from build123d import *

# Parameters (mm, degrees)
BOSS_EXTRU_3_DEPTH = 2
BOSS_EXTRU_4_DEPTH = 19.3
ESQUISSE4_W        = 2
ESQUISSE4_H        = 18.565
ESQUISSE4_H_2      = 18.45
BOSS_EXTRU_5_DEPTH = 3.9
ESQUISSE5_W        = 4
ESQUISSE5_H        = 4
ESQUISSE5_R        = 1.15
ESQUISSE5_W_2      = 3.87
ESQUISSE5_H_2      = 3.3
BOSS_EXTRU_6_DEPTH = 5.7


with BuildPart() as part:
    # Esquisse1 → Boss.-Extru.3 (new body)
    with BuildSketch(Plane.XY):
        with BuildLine():
            Line((-70, 0), (-10.000000065, 0))
            ThreePointArc((-10.000000065, 0), (-2.928932211, 2.928932165), (0, 10))
            Line((0, 10), (0, 110))
            ThreePointArc((0, 110), (-2.928932188, 117.071067812), (-10, 120))
            Line((-10, 120), (-70, 120))
            ThreePointArc((-70, 120), (-77.071067812, 117.071067812), (-80, 110))
            Line((-80, 110), (-80, 10))
            ThreePointArc((-80, 10), (-77.071067812, 2.928932188), (-70, 0))
        make_face()
    extrude(amount=BOSS_EXTRU_3_DEPTH)

    # Esquisse3 → Boss.-Extru.4 (add)
    with BuildSketch(Plane.XY.offset(2)):
        with BuildLine():
            ThreePointArc((-80, 10), (-79.486832981, 6.83772234), (-78, 4))
            Line((-78, 4), (-78, 10))
            Line((-78, 10), (-78, 16))
            ThreePointArc((-78, 16), (-79.486832981, 13.16227766), (-80, 10))
        make_face()
        with BuildLine():
            ThreePointArc((-78, 4), (-77.071067812, 2.928932188), (-76, 2))
            Line((-76, 2), (-70, 2))
            ThreePointArc((-70, 2), (-75.656854249, 4.343145751), (-78, 10))
            Line((-78, 10), (-78, 4))
        make_face()
        with BuildLine():
            ThreePointArc((-76, 2), (-73.16227766, 0.513167019), (-70, 0))
            ThreePointArc((-70, 0), (-66.83772234, 0.513167019), (-64, 2))
            Line((-64, 2), (-70, 2))
            Line((-70, 2), (-76, 2))
        make_face()
        with BuildLine():
            Line((-70, 0), (-10, 0))
            ThreePointArc((-10, 0), (-13.16227766, 0.513167019), (-16, 2))
            Line((-16, 2), (-64, 2))
            ThreePointArc((-64, 2), (-66.83772234, 0.513167019), (-70, 0))
        make_face()
        with BuildLine():
            ThreePointArc((-80, 10), (-79.486832981, 13.16227766), (-78, 16))
            Line((-78, 16), (-78, 104))
            ThreePointArc((-78, 104), (-79.486832981, 106.83772234), (-80, 110))
            Line((-80, 110), (-80, 10))
        make_face()
        with BuildLine():
            ThreePointArc((-80, 110), (-79.486832981, 106.83772234), (-78, 104))
            Line((-78, 104), (-78, 110))
            Line((-78, 110), (-78, 116))
            ThreePointArc((-78, 116), (-79.486832981, 113.16227766), (-80, 110))
        make_face()
        with BuildLine():
            ThreePointArc((-78, 110), (-75.656854249, 115.656854249), (-70, 118))
            Line((-70, 118), (-76, 118))
            ThreePointArc((-76, 118), (-77.071067812, 117.071067812), (-78, 116))
            Line((-78, 116), (-78, 110))
        make_face()
        with BuildLine():
            Line((-70, 118), (-64, 118))
            ThreePointArc((-64, 118), (-66.83772234, 119.486832981), (-70, 120))
            ThreePointArc((-70, 120), (-73.16227766, 119.486832981), (-76, 118))
            Line((-76, 118), (-70, 118))
        make_face()
        with BuildLine():
            Line((-64, 118), (-16, 118))
            ThreePointArc((-16, 118), (-13.16227766, 119.486832981), (-10, 120))
            Line((-10, 120), (-70, 120))
            ThreePointArc((-70, 120), (-66.83772234, 119.486832981), (-64, 118))
        make_face()
        with BuildLine():
            ThreePointArc((-10, 120), (-13.16227766, 119.486832981), (-16, 118))
            Line((-16, 118), (-10, 118))
            Line((-10, 118), (-4, 118))
            ThreePointArc((-4, 118), (-6.83772234, 119.486832981), (-10, 120))
        make_face()
        with BuildLine():
            Line((-2, 110), (-2, 116))
            ThreePointArc((-2, 116), (-2.928932188, 117.071067812), (-4, 118))
            Line((-4, 118), (-10, 118))
            ThreePointArc((-10, 118), (-4.343145751, 115.656854249), (-2, 110))
        make_face()
        with BuildLine():
            ThreePointArc((-2, 104), (-0.513167019, 106.83772234), (0, 110))
            ThreePointArc((0, 110), (-0.513167019, 113.16227766), (-2, 116))
            Line((-2, 116), (-2, 110))
            Line((-2, 110), (-2, 104))
        make_face()
        with BuildLine():
            ThreePointArc((-2, 16), (-0.513167019, 13.16227766), (0, 10))
            Line((0, 10), (0, 110))
            ThreePointArc((0, 110), (-0.513167019, 106.83772234), (-2, 104))
            Line((-2, 104), (-2, 16))
        make_face()
        with BuildLine():
            Line((-2, 10), (-2, 4))
            ThreePointArc((-2, 4), (-0.513167019, 6.83772234), (0, 10))
            ThreePointArc((0, 10), (-0.513167019, 13.16227766), (-2, 16))
            Line((-2, 16), (-2, 10))
        make_face()
        with BuildLine():
            Line((-10, 2), (-4, 2))
            ThreePointArc((-4, 2), (-2.928932188, 2.928932188), (-2, 4))
            Line((-2, 4), (-2, 10))
            ThreePointArc((-2, 10), (-4.343145751, 4.343145751), (-10, 2))
        make_face()
        with BuildLine():
            ThreePointArc((-10, 0), (-6.83772234, 0.513167019), (-4, 2))
            Line((-4, 2), (-10, 2))
            Line((-10, 2), (-16, 2))
            ThreePointArc((-16, 2), (-13.16227766, 0.513167019), (-10, 0))
        make_face()
    extrude(amount=BOSS_EXTRU_4_DEPTH)

    # Esquisse4 → Boss.-Extru.5 (add)
    with BuildSketch(Plane.XY.offset(21.3)):
        with BuildLine():
            Line((-64, 118), (-16, 118))
            ThreePointArc((-16, 118), (-13.16227766, 119.486832981), (-10, 120))
            Line((-10, 120), (-70, 120))
            ThreePointArc((-70, 120), (-66.83772234, 119.486832981), (-64, 118))
        make_face()
        with BuildLine():
            Line((-70, 118), (-64, 118))
            ThreePointArc((-64, 118), (-66.83772234, 119.486832981), (-70, 120))
            ThreePointArc((-70, 120), (-77.071067812, 117.071067812), (-80, 110))
            ThreePointArc((-80, 110), (-79.486832981, 106.83772234), (-78, 104))
            Line((-78, 104), (-78, 110))
            ThreePointArc((-78, 110), (-75.656854249, 115.656854249), (-70, 118))
        make_face()
        with BuildLine():
            Line((-2, 110), (-2, 104))
            ThreePointArc((-2, 104), (-0.513167019, 106.83772234), (0, 110))
            ThreePointArc((0, 110), (-2.928932188, 117.071067812), (-10, 120))
            ThreePointArc((-10, 120), (-13.16227766, 119.486832981), (-16, 118))
            Line((-16, 118), (-10, 118))
            ThreePointArc((-10, 118), (-4.343145751, 115.656854249), (-2, 110))
        make_face()
        with BuildLine():
            Line((-2, 104), (-2, 79.7))
            Line((-2, 79.7), (0, 79.7))
            Line((0, 79.7), (0, 110))
            ThreePointArc((0, 110), (-0.513167019, 106.83772234), (-2, 104))
        make_face()
        with Locations((-1, 62.8175)):
            Rectangle(ESQUISSE4_W, ESQUISSE4_H)
        with Locations((-1, 36.51)):
            Rectangle(ESQUISSE4_W, ESQUISSE4_H_2)
        with BuildLine():
            Line((0, 19.485), (-2, 19.485))
            Line((-2, 19.485), (-2, 16))
            ThreePointArc((-2, 16), (-0.513167019, 13.16227766), (0, 10))
            Line((0, 10), (0, 19.485))
        make_face()
        with BuildLine():
            ThreePointArc((0, 10), (-0.513167019, 13.16227766), (-2, 16))
            Line((-2, 16), (-2, 10))
            ThreePointArc((-2, 10), (-4.343145751, 4.343145751), (-10, 2))
            Line((-10, 2), (-16, 2))
            ThreePointArc((-16, 2), (-13.16227766, 0.513167019), (-10, 0))
            ThreePointArc((-10, 0), (-2.928932188, 2.928932188), (0, 10))
        make_face()
        with BuildLine():
            ThreePointArc((-64, 2), (-66.83772234, 0.513167019), (-70, 0))
            Line((-70, 0), (-10, 0))
            ThreePointArc((-10, 0), (-13.16227766, 0.513167019), (-16, 2))
            Line((-16, 2), (-64, 2))
        make_face()
        with BuildLine():
            ThreePointArc((-78, 16), (-79.486832981, 13.16227766), (-80, 10))
            ThreePointArc((-80, 10), (-77.071067812, 2.928932188), (-70, 0))
            ThreePointArc((-70, 0), (-66.83772234, 0.513167019), (-64, 2))
            Line((-64, 2), (-70, 2))
            ThreePointArc((-70, 2), (-75.656854249, 4.343145751), (-78, 10))
            Line((-78, 10), (-78, 16))
        make_face()
        with BuildLine():
            ThreePointArc((-78, 104), (-79.486832981, 106.83772234), (-80, 110))
            Line((-80, 110), (-80, 10))
            ThreePointArc((-80, 10), (-79.486832981, 13.16227766), (-78, 16))
            Line((-78, 16), (-78, 104))
        make_face()
    extrude(amount=BOSS_EXTRU_5_DEPTH)

    # Esquisse5 → Boss.-Extru.6 (add)
    # profile 1 of 4: a face of its own
    with BuildSketch(Plane.XY.offset(2)):
        with Locations((-4, 12)):
            Rectangle(ESQUISSE5_W, ESQUISSE5_H)
        with Locations((-4, 12)):
            Circle(ESQUISSE5_R, mode=Mode.SUBTRACT)
    # profile 2 of 4: a face of its own
    with BuildSketch(Plane.XY.offset(2)):
        with Locations((-60, 12)):
            Rectangle(ESQUISSE5_W, ESQUISSE5_H)
        with Locations((-60, 12)):
            Circle(ESQUISSE5_R, mode=Mode.SUBTRACT)
    # profile 3 of 4: a face of its own
    with BuildSketch(Plane.XY.offset(2)):
        with Locations((-60.065, 87.3)):
            Rectangle(ESQUISSE5_W_2, ESQUISSE5_H)
        with Locations((-60.065, 87.3)):
            Circle(ESQUISSE5_R, mode=Mode.SUBTRACT)
    # profile 4 of 4: a face of its own
    with BuildSketch(Plane.XY.offset(2)):
        with Locations((-4, 87.65)):
            Rectangle(ESQUISSE5_W, ESQUISSE5_H_2)
        with Locations((-4, 87.65)):
            Circle(ESQUISSE5_R, mode=Mode.SUBTRACT)
    extrude(amount=BOSS_EXTRU_6_DEPTH)


solid = part.part
Read the model definition and answer for the solid it produces. Units are mm, in the model's axes. A direction names the side the tool comes from. Give positions to 0.01 mm unless a question says otherwise; leave off trailing zeros. Write each loop counter-clockwise with the first axis right and the second up, starting at its lowest first coordinate (ties: lowest second). Pieces come first, ordered by that corner, then holes. Notation, with made-up numbers: (54, -22) - (72, -22) arc R27 ccw to (72, 5) - close; hole circle Ø3 at (-29, 89.25). An arc over 180 degrees is marked (long way). Answer in a Markdown table with one row per item. Add a question column.
Item 1: Flat-ended cylindrical pins translate along their axes: P1, Ø2, axis at x = -0.5, y = 24.5, coming from the +Z side; P2, Ø1.6, axis at x = -1, z = 23, coming from the -Y side; P3, Ø1.5, axis at x = -65.5, y = 107, coming from the +Z side. Find the tip coordinate at first contact, or state that the pin passes through.
Item 2: Section B-B, the plane z = 5 is taken. Count the separate pieces of the cut face and the enclosed holes in it, and give its area (3 significant figures).
Item 3: Section D-D, the plane x = -27.5 is taken. Write down the section's boundary in (y, z), and give its area (3 significant figures).
Item 4: Find the intervals of material crossed by L1, parallel to Y at x = -58.5, z = 4.5; L2, parallel to Y at x = -45, z = 14; L3, parallel to X at y = 40, z = 12.25, in increasing order.
Item 5: Section C-C, the plane y = 99.5 is taken. Write down the section's boundary in (x, z), and give its area (3 significant figures).
Item 6: A tool of negligible diameter and unlimited length cuts with its end or side. For faces 1 (the face through (-4.91, 11.3, 4.81)), 2 (the face through (-40, 120, 12)), from which of +Z, -Z, +X, -X, +Y, -Y can it reach the whole face along a straight path? Write none if from no direction.
Item 7: Section A-A, the plane z = 11.5 is taken. Write down the section's boundary in (x, y), and give its area (3 significant figures).
Item 8: Determine the mould class of faces 3 (the face through (-59.45, 88.27, 4.81)), 4 (the face through (-80, 61, 12)), 5 (the face through (-40, 0, 12)) for opening direction X: pulls with the +X half, pulls with the -X half, needs draft (parallel to the pull), parting line crosses it, or undercut.
Recorded:
| question | item | result |
|---|---|---|
| 1 | P1 | stops at z = 21.3 |
| 1 | P2 | stops at y = 4.28 |
| 1 | P3 | stops at z = 2 |
| 2 | separate pieces | 3 |
| 2 | enclosed holes | 5 |
| 2 | area | 797 mm2 |
| 3 | outline | (0, 0) - (120, 0) - (120, 25.2) - (118, 25.2) - (118, 2) - (2, 2) - (2, 25.2) - (0, 25.2) - close |
| 3 | area | 333 mm2 |
| 4 | L1 | y = 0 to 2, 10 to 14, 85.3 to 89.3, 118 to 120 |
| 4 | L2 | y = 0 to 2, 118 to 120 |
| 4 | L3 | x = -80 to -78, -2 to 0 |
| 5 | outline | (-80, 0) - (0, 0) - (0, 25.2) - (-2, 25.2) - (-2, 2) - (-78, 2) - (-78, 25.2) - (-80, 25.2) - close |
| 5 | area | 253 mm2 |
| 6 | face 1 | +Z |
| 6 | face 2 | +Z, -Z, +X, -X, +Y |
| 7 | outline | (-80, 10) arc R10 ccw to (-70, 0) - (-10, 0) arc R10 ccw to (0, 10) - (0, 110) arc R10 ccw to (-10, 120) - (-70, 120) arc R10 ccw to (-80, 110) - close; hole (-78, 10) arc R8 ccw to (-70, 2) - (-10, 2) arc R8 ccw to (-2, 10) - (-2, 110) arc R8 ccw to (-10, 118) - (-70, 118) arc R8 ccw to (-78, 110) - close |
| 7 | area | 753 mm2 |
| 8 | face 3 | undercut |
| 8 | face 4 | pulls with the -X half |
| 8 | face 5 | needs draft |
